Read the model definition and answer for the solid it produces. Units are mm, in the model's axes. Face numbers are marked on the shaded views. A direction names the side the tool comes from. Round coordinates to 2 decimals unless told otherwise and drop trailing zeros. Write each loop counter-clockwise with the first axis right and the second up, starting at its lowest first coordinate (ties: lowest second). Pieces come first, ordered by that corner, then holes.
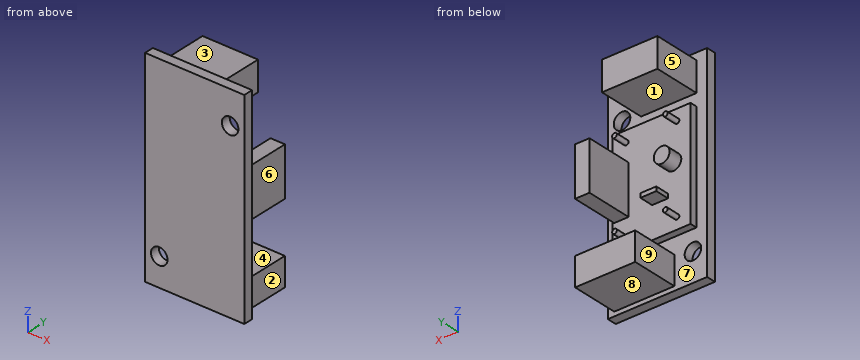
Autodesk Inventor part; units mm, degrees
ref_plane "YZ Plane" through (0, 0, 0) normal (1, 0, 0) x (0, 1, 0)
ref_plane "XZ Plane" through (0, 0, 0) normal (0, 1, 0) x (-1, 0, 0)
ref_plane "XY Plane" through (0, 0, 0) normal (0, 0, 1) x (1, 0, 0)
sketch "Szkic1" plane through (0, 0, 0) normal (0, 1, 0) x (-1, 0, 0)
  line L0 (-10.5, -21.75) -> (10.5, -21.75)
  line L1 (10.5, -21.75) -> (10.5, 21.75)
  line L2 (10.5, 21.75) -> (-10.5, 21.75)
  line L3 (-10.5, 21.75) -> (-10.5, -21.75)
  line L4 (-10.5, -21.75) -> (10.5, 21.75) construction
  line L5 (10.5, -21.75) -> (-10.5, 21.75) construction
  point P0 (0, 0)
  dimension "d0" = 21
  dimension "d1" = 43.5
extrude "Wyciągnięcie proste1" add sketch "Szkic1" along normal blind 2
sketch "Szkic2" plane through (0, 2, 0) normal (0, 1, 0) x (1, 0, 0)
  line L0 (-10.5, 21.75) -> (-10.5, -21.75)
  line L1 (-10.5, -21.75) -> (10.5, -21.75)
  line L2 (10.5, 21.75) -> (-10.5, 21.75)
  line L3 (10.5, -21.75) -> (10.5, 21.75)
  line L4 (0, 21.75) -> (0, -21.75)
  point P0 (0, 0)
  point P1 (7.5, -14.75)
  point P2 (-7.5, 15.75)
  dimension "d40" = 10.5
  dimension "d41" = 10.5
hole "Otwór1" at (7.5, 2, 14.75) at (-7.5, 2, -15.75) direction (0, -1, 0) diameter 3.5 end through all
sketch "Szkic3" plane through (0, 2, 0) normal (0, 1, 0) x (1, 0, 0)
  line L0 (8.25, 11.5) -> (-8.25, 11.5)
  line L1 (-8.25, 11.5) -> (-8.25, -11.5)
  line L2 (-8.25, -11.5) -> (8.25, -11.5)
  line L3 (8.25, -11.5) -> (8.25, 11.5)
  line L4 (8.25, 11.5) -> (-8.25, -11.5) construction
  line L5 (-8.25, 11.5) -> (8.25, -11.5) construction
  point P0 (0, 0)
  dimension "d15" = 16.5
  dimension "d16" = 23
extrude "Wyciągnięcie proste2" add sketch "Szkic3" along normal blind 1.5
sketch "Szkic4" plane through (0, 3.5, 0) normal (0, 1, 0) x (1, 0, 0)
  line L0 (8.25, 11.5) -> (-8.25, 11.5)
  line L1 (-8.25, 11.5) -> (-8.25, -11.5)
  line L2 (-8.25, -11.5) -> (8.25, -11.5)
  line L3 (8.25, -11.5) -> (8.25, 11.5)
  circle A0 centre (-5.375, -9.1) radius 0.5
  circle A1 centre (5.375, -9.1) radius 0.5
  circle A2 centre (5.375, 9.1) radius 0.5
  circle A3 centre (-5.375, 9.1) radius 0.5
  circle A4 centre (-4.6129, -1.6011) radius 1.6664
  line L4 (-0.1119, 4.829) -> (-3.4753, 4.829)
  line L5 (-3.4753, 4.829) -> (-3.4753, 3.9387)
  line L6 (-3.4753, 3.9387) -> (-0.1119, 3.9387)
  line L7 (-0.1119, 3.9387) -> (-0.1119, 4.829)
  line L8 (-0.1119, 4.829) -> (-3.4753, 3.9387) construction
  line L9 (-3.4753, 4.829) -> (-0.1119, 3.9387) construction
  point P0 (0, 0)
  point P1 (-1.7936, 4.3838)
  dimension "d19" = 10.75
  dimension "d20" = 10.75
  dimension "d21" = 2.875
  dimension "d22" = 2.875
  dimension "d23" = 2.875
  dimension "d24" = 2.875
  dimension "d25" = 18.2
  dimension "d26" = 18.2
  dimension "d27" = 2.4
  dimension "d28" = 2.4
  dimension "d29" = 2.4
  dimension "d30" = 1
  dimension "d31" = 1
  dimension "d32" = 1
  dimension "d33" = 1
extrude "Wyciągnięcie proste3" add sketch "Szkic4" along normal blind 3 contours A0 | A1 | A2 | A3 | A4 | L7 L6 L5 L4
sketch "Szkic5" plane through (0, 3.5, 0) normal (0, 1, 0) x (1, 0, 0)
  line L0 (-0.1119, 4.829) -> (-0.1119, 3.9387)
  line L1 (-0.1119, 3.9387) -> (-3.4753, 3.9387)
  line L2 (-3.4753, 3.9387) -> (-3.4753, 4.829)
  line L3 (-3.4753, 4.829) -> (-0.1119, 4.829)
  circle A0 centre (5.375, 9.1) radius 0.5
  circle A1 centre (-5.375, -9.1) radius 0.5
  circle A2 centre (5.375, -9.1) radius 0.5
  circle A3 centre (-5.375, 9.1) radius 0.5
  circle A4 centre (-4.6129, -1.6011) radius 1.6664
  line L4 (8.25, 11.5) -> (-8.25, 11.5)
  line L5 (-8.25, 11.5) -> (-8.25, -11.5)
  line L6 (-8.25, -11.5) -> (8.25, -11.5)
  line L7 (8.25, -11.5) -> (8.25, 11.5)
  line L8 (7.9153, 5.177) -> (4.875, 5.177)
  line L9 (4.875, 5.177) -> (4.875, -5.177)
  line L10 (4.875, -5.177) -> (7.9153, -5.177)
  line L11 (7.9153, -5.177) -> (7.9153, 5.177)
  line L12 (7.9153, 5.177) -> (4.875, -5.177) construction
  line L13 (4.875, 5.177) -> (7.9153, -5.177) construction
  point P0 (0, 0)
  point P1 (6.3951, 0)
extrude "Wyciągnięcie proste4" add sketch "Szkic5" along normal blind 10 contours L11 L10 L9 L8
sketch "Szkic6" plane through (0, 2, 0) normal (0, 1, 0) x (1, 0, 0)
  line L0 (7.9153, 5.177) -> (7.9153, -5.177)
  line L1 (7.9153, -5.177) -> (4.875, -5.177)
  line L2 (4.875, -5.177) -> (4.875, 5.177)
  line L3 (4.875, 5.177) -> (7.9153, 5.177)
  line L4 (-0.1119, 4.829) -> (-0.1119, 3.9387)
  line L5 (-0.1119, 3.9387) -> (-3.4753, 3.9387)
  line L6 (-3.4753, 3.9387) -> (-3.4753, 4.829)
  line L7 (-3.4753, 4.829) -> (-0.1119, 4.829)
  circle A0 centre (5.375, 9.1) radius 0.5
  circle A1 centre (-5.375, -9.1) radius 0.5
  circle A2 centre (5.375, -9.1) radius 0.5
  circle A3 centre (-5.375, 9.1) radius 0.5
  circle A4 centre (-4.6129, -1.6011) radius 1.6664
  line L8 (8.25, 11.5) -> (-8.25, 11.5)
  line L9 (-8.25, 11.5) -> (-8.25, -11.5)
  line L10 (-8.25, -11.5) -> (8.25, -11.5)
  line L11 (8.25, -11.5) -> (8.25, 11.5)
  line L12 (3.4647, -14.0449) -> (-8.2686, -14.0449)
  line L13 (-8.2686, -14.0449) -> (-8.2686, -20.2659)
  line L14 (-8.2686, -20.2659) -> (3.4647, -20.2659)
  line L15 (3.4647, -20.2659) -> (3.4647, -14.0449)
  line L16 (3.4647, -14.0449) -> (-8.2686, -20.2659) construction
  line L17 (-8.2686, -14.0449) -> (3.4647, -20.2659) construction
  line L18 (9.146, 20.8464) -> (-3.5644, 20.8464)
  line L19 (-3.5644, 20.8464) -> (-3.5644, 14.8558)
  line L20 (-3.5644, 14.8558) -> (9.146, 14.8558)
  line L21 (9.146, 14.8558) -> (9.146, 20.8464)
  line L22 (9.146, 20.8464) -> (-3.5644, 14.8558) construction
  line L23 (-3.5644, 20.8464) -> (9.146, 14.8558) construction
  point P0 (0, 0)
  point P1 (-2.4019, -17.1554)
  point P2 (2.7908, 17.8511)
extrude "Wyciągnięcie proste5" add sketch "Szkic6" along normal blind 10 contours L15 L14 L13 L12 | L21 L20 L19 L18
properties part number "step down"
Q1. Section B-B (z = -15.75) is taken. Determine the outline of the cut face in (x, y), then the cut area to 3 significant figures.
Verdict:
outline: (-10.5, 0) - (-9.25, 0) - (-9.25, 2) - (-10.5, 2) - close; (-5.75, 0) - (10.5, 0) - (10.5, 2) - (9.15, 2) - (9.15, 12) - (-3.56, 12) - (-3.56, 2) - (-5.75, 2) - close
area: 162 mm2
Q2. Determine the mould class of the marked faces 1, 2, 3 and 4 for opening direction Z: pulls with the +Z half, pulls with the -Z half, needs draft (parallel to the pull), parting line crosses it, or undercut.
Verdict:
face 1: undercut
face 2: needs draft
face 3: pulls with the +Z half
face 4: undercut
Q3. Which of the six approach directions +Z, -Z, +X, -X, +Y, -Y give full straight-line access (tool end or side, diameter ignored) to the marked faces 5, 6, 7, 8 and 9?
Verdict:
face 5: +Z, -Z, -X, +Y
face 6: +Z, +X, +Y
face 7: +Y
face 8: -Z, +X, -X, +Y
face 9: -Z, -X, +Y
Q4. Section A-A (x = -7.5) is taken. Determine the outline of the cut face in (y, z), then the cut area to 3 significant figures.
Verdict:
outline: (0, -21.75) - (2, -21.75) - (2, -17.5) - (0, -17.5) - close; (0, -14) - (2, -14) - (2, -11.5) - (3.5, -11.5) - (3.5, 11.5) - (2, 11.5) - (2, 14.04) - (12, 14.04) - (12, 20.27) - (2, 20.27) - (2, 21.75) - (0, 21.75) - close
area: 177 mm2
Q5. Section C-C (y = 5) is taken. State how many separate pieces and enclosed holes the cut face has, then the cut area to 3 significant figures.
Verdict:
separate pieces: 9
enclosed holes: 0
area: 195 mm2
Q6. Flat-ended cylindrical pins translate along their axes: pin 1 Ø3 at (x, z) = (0, 1.5) entering from +Y; pin 2 Ø3 at (x, z) = (-5, 18.5) entering from +Y; pin 3 Ø5 at (x, z) = (8.5, 1.5) entering from +Y; pin 4 Ø1.5 at (y, z) = (12, 12) entering from -X. Find the tip coordinate at first contact, or state that the pin passes through.
Verdict:
pin 1: stops at y = 3.5
pin 2: stops at y = 12
pin 3: stops at y = 13.5
pin 4: passes through
Q7. Section D-D (x = 1.5) is taken. Determine the outline of the cut face in (y, z), then the cut area to 3 significant figures.
Verdict:
outline: (0, -21.75) - (2, -21.75) - (2, -20.85) - (12, -20.85) - (12, -14.86) - (2, -14.86) - (2, -11.5) - (3.5, -11.5) - (3.5, 11.5) - (2, 11.5) - (2, 14.04) - (12, 14.04) - (12, 20.27) - (2, 20.27) - (2, 21.75) - (0, 21.75) - close
area: 244 mm2
Q8. Straight lines are drawn through the part: probe 1 along Z at (x, y) = (3.25, 7.5); probe 2 along X at (y, z) = (1.5, -15.75); probe 3 along Z at (x, y) = (-5.5, 5.5). For each, find the intervals that lie inside material, in ascending order.
Verdict:
probe 1: z = -20.85 to -14.86, 14.04 to 20.27
probe 2: x = -10.5 to -9.25, -5.75 to 10.5
probe 3: z = -9.58 to -8.62, 0.19 to 3.01, 8.62 to 9.58, 14.04 to 20.27
